```python
from build123d import *

# Parameters (mm, degrees)
F1_W     = 25.3
F1_H     = 3.2
F1_R     = 1.55
F1_W_2   = 3.2
F1_H_2   = 10.3
F2_DEPTH = 3.2
F3_R     = 5


with BuildPart() as f2:
    # F1 (on Front) → F2 (new body)
    with BuildSketch(Plane.XZ):
        Polygon((-99, 81), (-103, 81), (-103, 0), (-99, 0), (99, 0), (103, 0), (103, 81), (99, 81), align=None)
        with Locations((-75, 11.6)):
            Rectangle(F1_W, F1_H, mode=Mode.SUBTRACT)
        with Locations((-37.5, 11.6)):
            Circle(F1_R, mode=Mode.SUBTRACT)
        with Locations((0, 11.6)):
            Rectangle(F1_W, F1_H, mode=Mode.SUBTRACT)
        with Locations((-97.4, 23)):
            Rectangle(F1_W_2, F1_H_2, mode=Mode.SUBTRACT)
        with Locations((37.5, 11.6)):
            Circle(F1_R, mode=Mode.SUBTRACT)
        with Locations((75, 11.6)):
            Rectangle(F1_W, F1_H, mode=Mode.SUBTRACT)
        with Locations((97.4, 23)):
            Rectangle(F1_W_2, F1_H_2, mode=Mode.SUBTRACT)
        with Locations((-97.4, 40.5)):
            Circle(F1_R, mode=Mode.SUBTRACT)
        with Locations((-97.4, 58)):
            Rectangle(F1_W_2, F1_H_2, mode=Mode.SUBTRACT)
        with Locations((-75, 69.4)):
            Rectangle(F1_W, F1_H, mode=Mode.SUBTRACT)
        with Locations((-37.5, 69.4)):
            Circle(F1_R, mode=Mode.SUBTRACT)
        with Locations((0, 69.4)):
            Rectangle(F1_W, F1_H, mode=Mode.SUBTRACT)
        with Locations((97.4, 40.5)):
            Circle(F1_R, mode=Mode.SUBTRACT)
        with Locations((97.4, 58)):
            Rectangle(F1_W_2, F1_H_2, mode=Mode.SUBTRACT)
        with Locations((37.5, 69.4)):
            Circle(F1_R, mode=Mode.SUBTRACT)
        with Locations((75, 69.4)):
            Rectangle(F1_W, F1_H, mode=Mode.SUBTRACT)
    extrude(amount=F2_DEPTH)

    # F3
    f3_edges = [f2.edges().sort_by_distance(p)[0] for p in [
        (-103, -1.6, 81),
        (-103, -1.6, 0),
        (103, -1.6, 81),
        (103, -1.6, 0),
    ]]
    fillet(f3_edges, radius=F3_R)


solid = f2.part
```
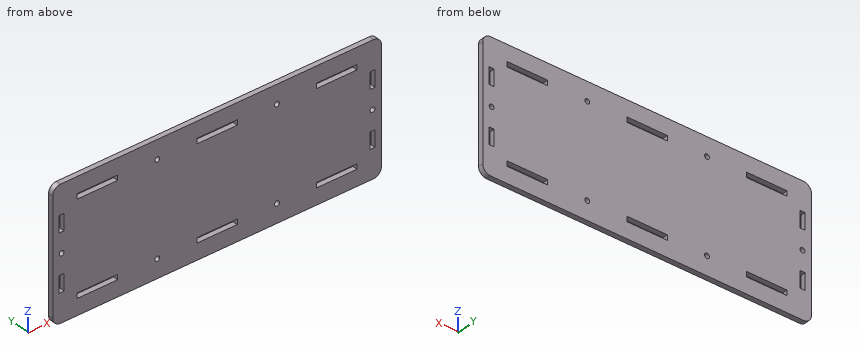
The listing builds one solid part. Answer for the finished solid, in the listing's coordinates (mm). Give positions to 0.01 mm unless a question says otherwise; leave off trailing zeros. Order: outer loops, then holes, each group sorted by start corner. A loop starts at its lowest first (then second) coordinate and runs counter-clockwise, first axis right, second up. Notation, with made-up numbers: (55.25, 30) -> (67.25, 30) arc R17 ccw to (67.25, 63) -> close; hole circle Ø6 at (56, 38.5). An arc over 180 degrees is marked (long way). Answer as CSV lines item,"result". Start each with the question number.
Q1. Find the intervals of material crossed by L1, parallel to X at y = -1, z = 26; L2, parallel to X at y = -1.6, z = 69.4; L3, parallel to Z at x = -64, y = -1.25, in increasing order.
Q2. A cutting plane is placed at A-A (x = -7). Determine the outline of the cut face in (y, z).
Q3. A cutting plane is placed at B-B (y = -0.85). Count the separate pieces of the cut face and the enclosed holes in it, then the cut area to 3 significant figures.
Results found:
1,L1,"-103 to -99, -95.8 to 95.8, 99 to 103"
1,L2,"-103 to -87.65, -62.35 to -39.05, -35.95 to -12.65, 12.65 to 35.95, 39.05 to 62.35, 87.65 to 103"
1,L3,"0 to 10, 13.2 to 67.8, 71 to 81"
2,outline,"(-3.2, 0) -> (0, 0) -> (0, 10) -> (-3.2, 10) -> close; (-3.2, 13.2) -> (0, 13.2) -> (0, 67.8) -> (-3.2, 67.8) -> close; (-3.2, 71) -> (0, 71) -> (0, 81) -> (-3.2, 81) -> close"
3,separate pieces,"1"
3,enclosed holes,"16"
3,area,"16,000 mm2"
